Study the drawing (mm; zero at the part's minimum x, y, z) and answer. Round coordinates to 2 decimals unless told otherwise and drop trailing zeros. Loops run counter-clockwise (first coordinate to the right, second up) from the corner with the lowest first, then second, coordinate; pieces in that order, holes last. Notation, with made-up numbers: (-33.75, 35.5) -> (13.25, 35.5) arc R27 ccw to (13.25, 56.5) -> close; hole circle Ø3 at (-29.75, -37.75). An arc over 180 degrees is marked (long way). Answer in a Markdown table with one row per item. Add a question column.
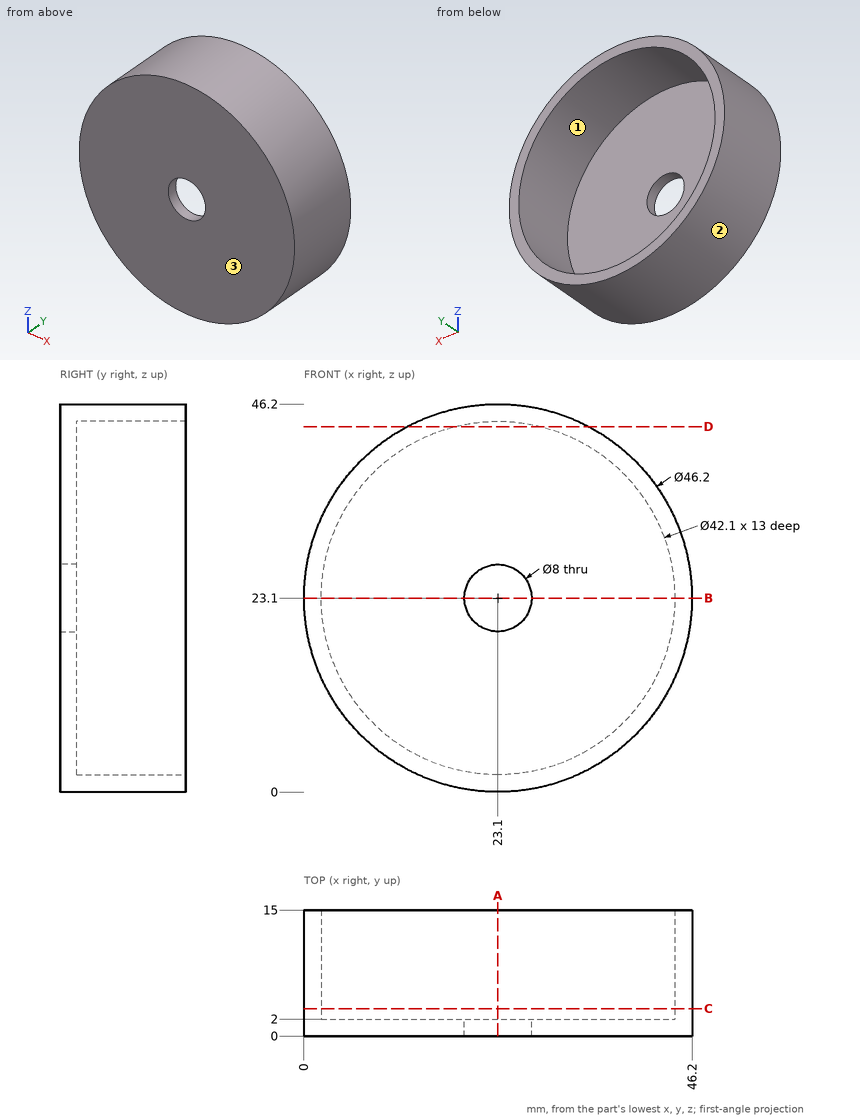
Item 1: The mould has two halves that part along Z. Classify the marked faces 1, 2 and 3: +Z half, -Z half, draft (parallel to the pull), parting line (faces both ways), or undercut.
Item 2: Section B-B, the plane z = 23.1 is taken. Write down the section's boundary in (x, y).
Item 3: Section A-A, the plane x = 23.1 is taken. Write down the section's boundary in (y, z), and give its area (3 significant figures).
Item 4: Flat-ended cylindrical pins translate along their axes: P1, Ø6, axis at x = 8.5, z = 27, coming from the -Y side; P2, Ø8, axis at y = 10.5, z = 18.5, coming from the +X side; P3, Ø1, axis at x = 7.5, z = 16, coming from the +Y side. Find the tip coordinate at first contact, or state that the pin passes through.
Item 5: Consider L1, parallel to X at y = 0.95, z = 23.1; L2, parallel to X at y = 5.75, z = 22.5; L3, parallel to Y at x = 41, z = 24.5. Determine where each line is inside the solid, lowest interval first. Write a range as from..to.
Item 6: Section D-D, the plane z = 43.5 is taken. Write down the section's boundary in (x, y), and give its area (3 significant figures).
Item 7: Section C-C, the plane y = 3.25 is taken. Write down the section's boundary in (x, z).
Here are the results:
| question | item | result |
|---|---|---|
| 1 | face 1 | undercut |
| 1 | face 2 | parting line |
| 1 | face 3 | draft |
| 2 | outline | (0, 0) -> (19.1, 0) -> (19.1, 2) -> (2.05, 2) -> (2.05, 15) -> (0, 15) -> close; (27.1, 0) -> (46.2, 0) -> (46.2, 15) -> (44.15, 15) -> (44.15, 2) -> (27.1, 2) -> close |
| 3 | outline | (0, 0) -> (15, 0) -> (15, 2.05) -> (2, 2.05) -> (2, 19.1) -> (0, 19.1) -> close; (0, 27.1) -> (2, 27.1) -> (2, 44.15) -> (15, 44.15) -> (15, 46.2) -> (0, 46.2) -> close |
| 3 | area | 130 mm² |
| 4 | P1 | stops at y = 0 |
| 4 | P2 | stops at x = 46.19 |
| 4 | P3 | stops at y = 2 |
| 5 | L1 | x = 0..19.1, 27.1..46.2 |
| 5 | L2 | x = 0.01..2.06, 44.14..46.19 |
| 5 | L3 | y = 0..2 |
| 6 | outline | (12.26, 0) -> (33.94, 0) -> (33.94, 15) -> (28.29, 15) -> (28.29, 2) -> (17.91, 2) -> (17.91, 15) -> (12.26, 15) -> close |
| 6 | area | 190 mm² |
| 7 | outline | circle Ø46.2 at (23.1, 23.1); hole circle Ø42.1 at (23.1, 23.1) |
